Could you check a few things on this drawing? It's one solid part, dimensions in mm from its lowest x, y, z. Coordinates: 2 decimals unless noted, no trailing zeros. Answer as a JSON object with one key per item and string values. Group by question number.
Item 1: We'd pull the mould along Y, two halves only. Please class the marked faces 1 and 2: +Y half, -Y half, draft (parallel to the pull), parting line (faces both ways), or undercut.
Item 2: I'm going to push a flat-ended pin straight in: pin 1 Ø20.5 at (x, z) = (21, 69) entering from +Y. Where does the tip first touch, or does it pass through?
Item 3: If I drill on line 1 (X direction, y = 2.25, z = 30); line 2 (Z direction, x = 5, y = 1.05); line 3 (X direction, y = 0.3, z = 82), over which ranges is the centre line in solid material (lowest first)?
Item 4: Suppose I cut it at C-C (z = 10). Count the separate pieces of the cut face and the enclosed holes in it, then the cut area to 3 significant figures.
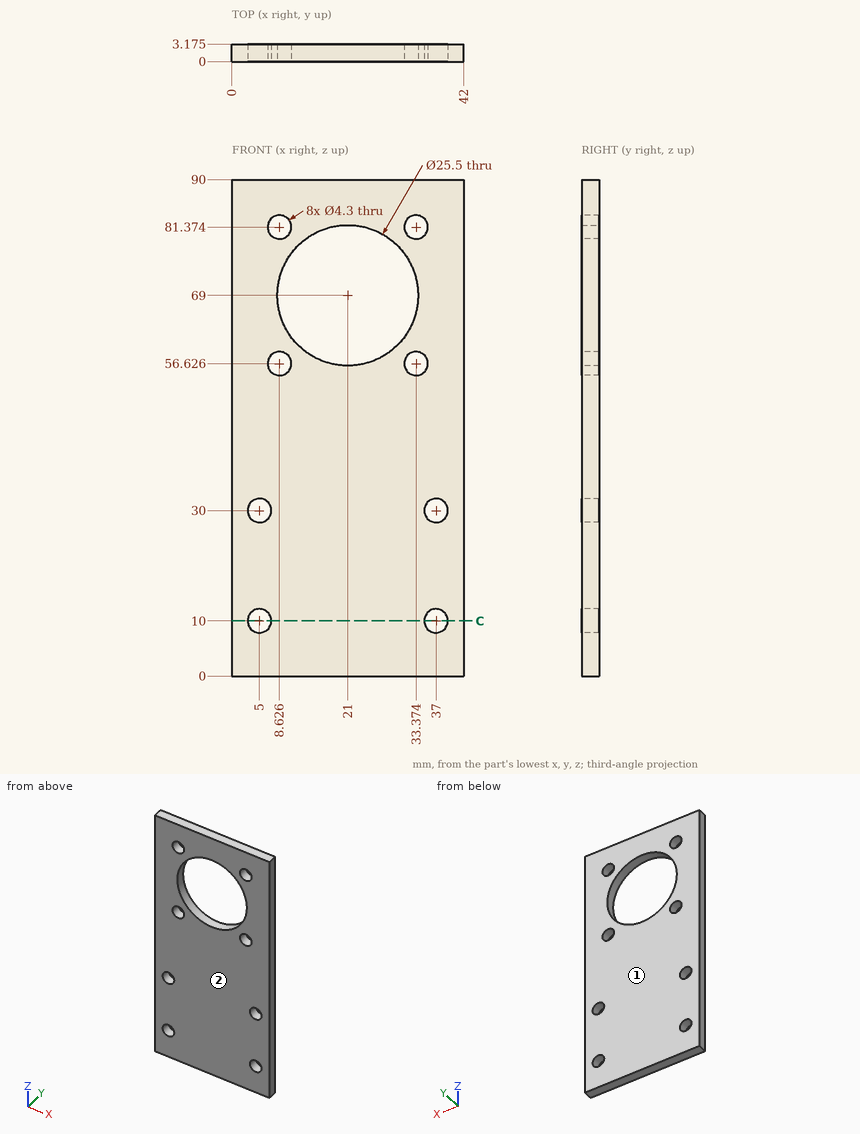
From the geometry:
{
 "1": {"face 1": "+Y half", "face 2": "-Y half"},
 "2": {"pin 1": "through"},
 "3": {"line 1": "0 to 2.85, 7.15 to 34.85, 39.15 to 42", "line 2": "0 to 7.85, 12.15 to 27.85, 32.15 to 90", "line 3": "0 to 6.57, 10.68 to 31.32, 35.43 to 42"},
 "4": {"separate pieces": "3", "enclosed holes": "0", "area": "106 mm2"}
}
